Source: CAD feature listing. Evaluate the final solid. Frame: model axes, mm. Face numbers are marked on the shaded views. A direction names the side the tool comes from. Coordinates: 2 decimals unless noted, no trailing zeros. Order: outer loops, then holes, each group sorted by start corner. A loop starts at its lowest first (then second) coordinate and runs counter-clockwise, first axis right, second up.
```python
from build123d import *

# Parameters (mm, degrees)
SKETCH1_W               = 130
SKETCH1_H               = 70
BOSS_EXTRUDE1_DEPTH     = 27
SKETCH2_R               = 1.75
CUT_EXTRUDE1_DEPTH      = 27
CUT_EXTRUDE2_START      = -21
CUT_EXTRUDE2_OUTLINE_R  = 1.75
CUT_EXTRUDE2_DEPTH      = 21
CUT_EXTRUDE3_DEPTH      = 100.823879977
CUT_EXTRUDE3_DEPTH_BACK = 100.823879977
CUT_EXTRUDE4_DEPTH      = 80.987499152
CUT_EXTRUDE4_DEPTH_BACK = 80.987499152
SKETCH5_R               = 1.65
SKETCH5_R_2             = 2.2
CUT_EXTRUDE5_DEPTH      = 2
FILLET2_R               = 8


# Read off the part's stored shape, not the designer's step: Cut-Extrude2
with BuildPart() as part:
    # Sketch1 → Boss-Extrude1 (new body)
    with BuildSketch(Plane(origin=(0, 0, 0), x_dir=(1, 0, 0), z_dir=(0, 1, 0))):
        Rectangle(SKETCH1_W, SKETCH1_H)
    extrude(amount=BOSS_EXTRUDE1_DEPTH)

    # Sketch2 → Cut-Extrude1 (cut)
    with BuildSketch(Plane(origin=(0, 27, 0), x_dir=(1, 0, 0), z_dir=(0, 1, 0))):
        with BuildLine():
            Line((65, 35), (-4, 35))
            add(Edge.make_bspline(
                [(16.985276193, 32.037400285), (16.344384253, 31.734586923), (15.139997676, 31.224413868), (13.363177927, 30.647367552), (11.717672063, 30.264833972), (10.188111987, 30.048519757), (8.761038737, 29.968698707), (7.386612758, 30.001896041), (6.043994999, 30.146954639), (4.647593927, 30.414660082), (3.19578664, 30.821123925), (1.740907748, 31.375111265), (0.506749671, 31.963769434), (-0.587741435, 32.566280044), (-1.628944852, 33.212844151), (-2.805878859, 34.038462463), (-3.58582038, 34.654179882), (-4, 35)],
                knots=[0, 0, 0, 0, 0.094281903, 0.173839808, 0.248204838, 0.318741989, 0.379062302, 0.438143998, 0.501439531, 0.558475445, 0.627109695, 0.701723198, 0.765277059, 0.808848652, 0.867872888, 0.928222089, 1, 1, 1, 1], degree=3))
            ThreePointArc((16.985276193, 32.037400285), (17.619352011, 32.111625453), (18.169122212, 31.787103892))
            add(Edge.make_bspline(
                [(18.169122212, 31.787103892), (18.880572219, 30.963826417), (20.353964659, 29.282877442), (22.960721292, 26.394523325), (25.956424204, 23.194668161), (29.413337423, 19.655492092), (32.721030959, 16.412362495), (36.121712054, 13.209386341), (40.056563488, 9.645356576), (46.199565364, 4.366442592), (51.289830213, 0.354927225), (54.600855171, -2.113733504)],
                knots=[0, 0, 0, 0, 0.065465906, 0.134483043, 0.234080041, 0.329168047, 0.432121818, 0.51276386, 0.610223282, 0.751517468, 1, 1, 1, 1], degree=3))
            ThreePointArc((54.600855171, -2.113733504), (55.000762083, -2.84691143), (54.704832326, -3.627873009))
            add(Edge.make_bspline(
                [(54.704832326, -3.627873009), (53.498966947, -4.81552915), (51.311897548, -7.140167952), (48.69963123, -10.367424816), (46.601925875, -13.292582874), (44.80812232, -16.078484523), (43.184554029, -18.939393608), (41.54418466, -22.201248931), (40.571491097, -24.44033411), (40.018197727, -25.840134095)],
                knots=[0, 0, 0, 0, 0.189281305, 0.356736472, 0.463941083, 0.591760781, 0.727143489, 0.83164987, 1, 1, 1, 1], degree=3))
            ThreePointArc((40.018197727, -25.840134095), (39.375842934, -26.43026519), (38.514642112, -26.291673943))
            Line((38.514642112, -26.291673943), (11.207024421, -7.170674209))
            add(Edge.make_bspline(
                [(-14, -8), (-12.271757293, -6.971672517), (-9.466063488, -5.598856445), (-5.386625364, -4.405667761), (-2.228024111, -3.944265665), (0.835893041, -3.933946272), (3.534272193, -4.284331997), (7.080143183, -5.174272804), (9.554008371, -6.255827229), (11.207024421, -7.170674209)],
                knots=[0, 0, 0, 0, 0.227553532, 0.351236087, 0.479384283, 0.587200541, 0.696804288, 0.786205014, 1, 1, 1, 1], degree=3))
            Line((-14, -8), (-34.5, -8))
            add(Edge.make_bspline(
                [(-34.5, -8), (-34.998716381, -6.018305789), (-35.964034069, -2.659544028), (-37.427398174, 1.315845087), (-38.863544091, 4.641999873), (-40.252890439, 7.393277622), (-42.354272337, 10.856052977), (-44.782138282, 14.09338159), (-47.910103128, 17.205621078), (-51.557866637, 19.931151613), (-55.480439434, 21.894814973), (-60.176202103, 23.297139891), (-63.196027982, 23.703049389), (-65, 23.797699279)],
                knots=[0, 0, 0, 0, 0.128897983, 0.220226627, 0.266962342, 0.357379422, 0.414326697, 0.522335212, 0.611659128, 0.691709781, 0.808709753, 0.886032473, 1, 1, 1, 1], degree=3))
            Line((-65, 23.797699279), (-65, -35))
            Line((-65, -35), (65, -35))
            Line((65, -35), (65, 35))
        make_face()
        Polygon((33.591106657, -17.961078948), (0.005872841, 5.555554943), (12.050978004, 22.757747873), (45.63621182, -0.758886018), align=None)
        with BuildLine():
            add(Edge.make_bspline(
                [(-12.50850871, 27), (-13.456798873, 24.573487755), (-14.814722597, 19.89522318), (-15.579858129, 12.089800552), (-15.057965095, 6.888745359), (-14.472989206, 4)],
                knots=[0, 0, 0, 0, 0.333751147, 0.622103639, 1, 1, 1, 1], degree=3))
            Line((-14.472989206, 4), (-26.5, 4))
            add(Edge.make_bspline(
                [(-45.563538233, 27), (-42.772339428, 25.689399679), (-38.343403879, 22.999001318), (-33.000298141, 17.764831394), (-28.975299715, 11.692876511), (-27.193040414, 6.790024988), (-26.5, 4)],
                knots=[0, 0, 0, 0, 0.299156058, 0.498403991, 0.72092627, 1, 1, 1, 1], degree=3))
            Line((-45.563538233, 27), (-12.50850871, 27))
        make_face()
        with Locations(Location((0.293511086, 12.068408714, 0), (0, 0, 270))):
            Circle(SKETCH2_R)
        with Locations(Location((6.029275449, 20.259929156, 0), (0, 0, 270))):
            Circle(SKETCH2_R)
        with Locations(Location((45.348573575, -7.271739788, 0), (0, 0, 270))):
            Circle(SKETCH2_R)
        with Locations(Location((39.612809212, -15.463260231, 0), (0, 0, 270))):
            Circle(SKETCH2_R)
    extrude(amount=-CUT_EXTRUDE1_DEPTH, mode=Mode.SUBTRACT)

    # Cut-Extrude2 outline → Cut-Extrude2 (cut)
    with BuildSketch(Plane(origin=(0, 27, 0), x_dir=(1, 0, 0), z_dir=(0, 1, 0)).offset(CUT_EXTRUDE2_START)):
        with BuildLine():
            add(Edge.make_bspline(
                [(-34.5, -8), (-34.998716381, -6.018305789), (-35.964034069, -2.659544028), (-37.427398174, 1.315845087), (-38.863544091, 4.641999873), (-40.252890439, 7.393277622), (-42.354272337, 10.856052977), (-44.782138282, 14.09338159), (-47.910103128, 17.205621078), (-51.557866637, 19.931151613), (-55.480439434, 21.894814973), (-60.176202103, 23.297139891), (-63.196027982, 23.703049389), (-65, 23.797699279)],
                knots=[0, 0, 0, 0, 0.128897983, 0.220226627, 0.266962342, 0.357379422, 0.414326697, 0.522335212, 0.611659128, 0.691709781, 0.808709753, 0.886032473, 1, 1, 1, 1], degree=3))
            Line((-34.5, -8), (-34.5, 0.3))
            Line((-34.5, 0.3), (-14, 0.3))
            Line((-14, 0.3), (-14, -8))
            add(Edge.make_bspline(
                [(-14, -8), (-12.271757293, -6.971672517), (-9.466063488, -5.598856445), (-5.386625364, -4.405667761), (-2.228024111, -3.944265665), (0.835893041, -3.933946272), (3.534272193, -4.284331997), (7.080143183, -5.174272804), (9.554008371, -6.255827229), (11.207024421, -7.170674209)],
                knots=[0, 0, 0, 0, 0.227553532, 0.351236087, 0.479384283, 0.587200541, 0.696804288, 0.786205014, 1, 1, 1, 1], degree=3))
            Line((11.207024421, -7.170674209), (38.514642112, -26.291673943))
            ThreePointArc((38.514642112, -26.291673943), (39.375842934, -26.43026519), (40.018197727, -25.840134095))
            add(Edge.make_bspline(
                [(54.704832326, -3.627873009), (53.498966947, -4.81552915), (51.311897548, -7.140167952), (48.69963123, -10.367424816), (46.601925875, -13.292582874), (44.80812232, -16.078484523), (43.184554029, -18.939393608), (41.54418466, -22.201248931), (40.571491097, -24.44033411), (40.018197727, -25.840134095)],
                knots=[0, 0, 0, 0, 0.189281305, 0.356736472, 0.463941083, 0.591760781, 0.727143489, 0.83164987, 1, 1, 1, 1], degree=3))
            ThreePointArc((54.704832326, -3.627873009), (55.000762083, -2.84691143), (54.600855171, -2.113733504))
            add(Edge.make_bspline(
                [(18.169122212, 31.787103892), (18.880572219, 30.963826417), (20.353964659, 29.282877442), (22.960721292, 26.394523325), (25.956424204, 23.194668161), (29.413337423, 19.655492092), (32.721030959, 16.412362495), (36.121712054, 13.209386341), (40.056563488, 9.645356576), (46.199565364, 4.366442592), (51.289830213, 0.354927225), (54.600855171, -2.113733504)],
                knots=[0, 0, 0, 0, 0.065465906, 0.134483043, 0.234080041, 0.329168047, 0.432121818, 0.51276386, 0.610223282, 0.751517468, 1, 1, 1, 1], degree=3))
            ThreePointArc((18.169122212, 31.787103892), (17.619352011, 32.111625453), (16.985276193, 32.037400285))
            add(Edge.make_bspline(
                [(16.985276193, 32.037400285), (16.344384253, 31.734586923), (15.139997676, 31.224413868), (13.363177927, 30.647367552), (11.717672063, 30.264833972), (10.188111987, 30.048519757), (8.761038737, 29.968698707), (7.386612758, 30.001896041), (6.043994999, 30.146954639), (4.647593927, 30.414660082), (3.19578664, 30.821123925), (1.740907748, 31.375111265), (0.506749671, 31.963769434), (-0.587741435, 32.566280044), (-1.628944852, 33.212844151), (-2.805878859, 34.038462463), (-3.58582038, 34.654179882), (-4, 35)],
                knots=[0, 0, 0, 0, 0.094281903, 0.173839808, 0.248204838, 0.318741989, 0.379062302, 0.438143998, 0.501439531, 0.558475445, 0.627109695, 0.701723198, 0.765277059, 0.808848652, 0.867872888, 0.928222089, 1, 1, 1, 1], degree=3))
            Line((-4, 35), (-4, 24))
            Line((-4, 24), (-7, 24))
            Line((-7, 24), (-7, 30))
            Line((-7, 30), (-14, 30))
            Line((-14, 30), (-14, 35))
            Line((-14, 35), (-55, 35))
            Line((-55, 35), (-55, 30))
            Line((-55, 30), (-62, 30))
            Line((-62, 30), (-62, 24))
            Line((-62, 24), (-65, 24))
            Line((-65, 24), (-65, 23.797699279))
        make_face()
        with Locations((39.612809212, -15.463260231)):
            Circle(CUT_EXTRUDE2_OUTLINE_R, mode=Mode.SUBTRACT)
        Polygon((45.63621182, -0.758886018), (33.591106657, -17.961078948), (0.005872841, 5.555554943), (12.050978004, 22.757747873), align=None, mode=Mode.SUBTRACT)
        with Locations((45.348573575, -7.271739788)):
            Circle(CUT_EXTRUDE2_OUTLINE_R, mode=Mode.SUBTRACT)
        with BuildLine():
            Line((-45.563538233, 27), (-12.50850871, 27))
            add(Edge.make_bspline(
                [(-12.50850871, 27), (-13.456798873, 24.573487755), (-14.814722597, 19.89522318), (-15.579858129, 12.089800552), (-15.057965095, 6.888745359), (-14.472989206, 4)],
                knots=[0, 0, 0, 0, 0.333751147, 0.622103639, 1, 1, 1, 1], degree=3))
            Line((-14.472989206, 4), (-26.5, 4))
            add(Edge.make_bspline(
                [(-45.563538233, 27), (-42.772339428, 25.689399679), (-38.343403879, 22.999001318), (-33.000298141, 17.764831394), (-28.975299715, 11.692876511), (-27.193040414, 6.790024988), (-26.5, 4)],
                knots=[0, 0, 0, 0, 0.299156058, 0.498403991, 0.72092627, 1, 1, 1, 1], degree=3))
        make_face(mode=Mode.SUBTRACT)
        with Locations((0.293511086, 12.068408714)):
            Circle(CUT_EXTRUDE2_OUTLINE_R, mode=Mode.SUBTRACT)
        with Locations((6.029275449, 20.259929156)):
            Circle(CUT_EXTRUDE2_OUTLINE_R, mode=Mode.SUBTRACT)
    extrude(amount=CUT_EXTRUDE2_DEPTH, mode=Mode.SUBTRACT)

    # Sketch4 → Cut-Extrude3 (cut, two sides: drawn at the far end of the back side and taken through both)
    with BuildSketch(Plane.ZY.offset(34.5).offset(-CUT_EXTRUDE3_DEPTH_BACK)):
        Polygon((-0.3, 27), (3, 27), (3, 9.3), (-0.3, 6), align=None)
        Polygon((-24, 27), (-30, 27), (-30, 18), (-24, 6), align=None)
    extrude(amount=CUT_EXTRUDE3_DEPTH + CUT_EXTRUDE3_DEPTH_BACK, mode=Mode.SUBTRACT)

    # Sketch5 → Cut-Extrude4 (cut, two sides: drawn at the far end of the back side and taken through both)
    with BuildSketch(Plane(origin=(0, 0, 3), x_dir=(-1, 0, 0), z_dir=(0, 0, -1)).offset(-CUT_EXTRUDE4_DEPTH_BACK)):
        with Locations((10.5, 21.5)):
            Circle(SKETCH5_R)
        with Locations((10.5, 11.5)):
            Circle(SKETCH5_R)
        with Locations((58.5, 21.5)):
            Circle(SKETCH5_R)
        with Locations((58.5, 11.5)):
            Circle(SKETCH5_R)
        with Locations(Location((24.25, 16.5, 0), (0, 0, 180))):
            Circle(SKETCH5_R_2)
    extrude(amount=CUT_EXTRUDE4_DEPTH + CUT_EXTRUDE4_DEPTH_BACK, mode=Mode.SUBTRACT)

    # Sketch6 → Cut-Extrude5 (cut)
    with BuildSketch(Plane(origin=(0, 0, 3), x_dir=(-1, 0, 0), z_dir=(0, 0, -1))):
        Polygon((26.386195996, 20.2), (22.113804004, 20.2), (19.977608008, 16.5), (22.113804004, 12.8), (26.386195996, 12.8), (28.522391992, 16.5), align=None)
    extrude(amount=-CUT_EXTRUDE5_DEPTH, mode=Mode.SUBTRACT)

    # Fillet2
    fillet2_edges = [part.edges().sort_by_distance(p)[0] for p in [
        (-65, 0, -29.398849639),
    ]]
    fillet(fillet2_edges, radius=FILLET2_R)


solid = part.part
```
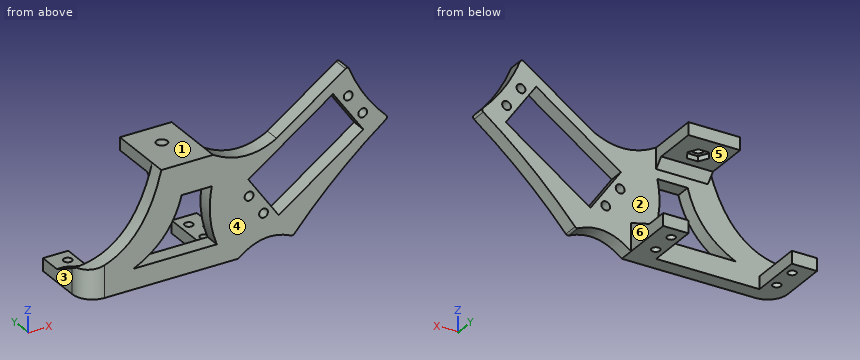
Q1. Section query A-A on y = 21.5. Output: boundary loops of the cut face in (x, z).
Solutions:
outline: (-65, -35) - (-60.15, -35) - (-60.15, -30) - (-65, -30) - close; (-56.85, -35) - (-55, -35) - (-55, -30) - (-56.85, -30) - close; (-34.5, 3) - (-14, 3) - (-14, 8) - (-34.5, 8) - close; (-14, -35) - (-12.15, -35) - (-12.15, -30) - (-14, -30) - close; (-8.85, -35) - (-4, -35) - (-4, -30) - (-8.85, -30) - close
Q2. Pull-direction query (X, two-part tool) for the marked faces 1, 2 and 3; classes: pulls with the +X half, pulls with the -X half, needs draft (parallel to the pull), parting line crosses it, or undercut.
Solutions:
face 1: needs draft
face 2: undercut
face 3: pulls with the -X half
Q3. Section query D-D on x = -10.5. Give the number of separate pieces and of enclosed holes in the cut face, plus the area to 3 significant figures.
Solutions:
separate pieces: 3
enclosed holes: 0
area: 319 mm2
Q4. Material intervals for line 1 along Y through (x, z) = (-10.5, -33.1); line 2 along X through (y, z) = (21.5, -32.7); line 3 along X through (y, z) = (16.5, 4), sorted ascending.
Solutions:
line 1: y = 0 to 9.85, 13.15 to 19.85, 23.15 to 27
line 2: x = -65 to -60.15, -56.85 to -55, -14 to -12.15, -8.85 to -4
line 3: x = -34.5 to -28.52, -19.98 to -14
Q5. Section query C-C on y = 11.5. Output: boundary loops of the cut face in (x, z), plus the area to 3 significant figures.
Solutions:
outline: (-65, -35) - (-60.15, -35) - (-60.15, -30) - (-62, -30) - (-62, -26.75) - (-65, -26.75) - close; (-56.85, -35) - (-55, -35) - (-55, -30) - (-56.85, -30) - close; (-34.5, 3) - (-14, 3) - (-14, 8) - (-34.5, 8) - close; (-14, -35) - (-12.15, -35) - (-12.15, -30) - (-14, -30) - close; (-8.85, -35) - (-4, -35) - (-4, -26.75) - (-7, -26.75) - (-7, -30) - (-8.85, -30) - close
area: 189 mm2
Q6. Pin query (flat end, axial travel): P1, Ø2.5, axis at y = 20.5, z = 5, coming from the +X side; P2, Ø18.5, axis at x = 4, z = 5.5, coming from the +Y side; P3, Ø5, axis at y = 8, z = 18, coming from the +X side. Return the tip coordinate at first contact, or that it passes through.
Solutions:
P1: stops at x = -14
P2: stops at y = 6
P3: stops at x = 44.59
Q7. Set-up query: the marked faces 4, 5 and 6. Return all of +Z, -Z, +X, -X, +Y, -Y with unobstructed straight access to the full face (end or side cutting, diameter ignored); none if empty.
Solutions:
face 4: +Z, -Z, +X, -X, -Y
face 5: -Z, +X, -X, +Y
face 6: +Z, -Z, +X, +Y
Q8. Section query B-B on x = -24.25. Output: boundary loops of the cut face in (y, z).
Solutions:
outline: (0, -35) - (6, -35) - (6, -27) - (0, -27) - close; (0, -4) - (6, -4) - (6, -0.3) - (9.3, 3) - (12.8, 3) - (12.8, 5) - (14.3, 5) - (14.3, 8) - (0, 8) - close; (18.7, 5) - (20.2, 5) - (20.2, 3) - (27, 3) - (27, 8) - (18.7, 8) - close
